from build123d import *

# Parameters (mm, degrees)
BOSS_EXTRUDE1_DEPTH = 29.972
CUT_EXTRUDE1_REACH  = 70.705
SKETCH2_R           = 19.939


with BuildPart() as part:
    # Sketch1 → Boss-Extrude1 (new body, symmetric)
    with BuildSketch(Plane.XY):
        Polygon((0, 0), (0, 59.944), (35.052, 59.944), (109.982, 0), align=None)
    extrude(amount=BOSS_EXTRUDE1_DEPTH, both=True)

    # Cut-Extrude1: up to this face of the body (flat: up to its plane)
    cut_extrude1_end = Plane(part.part.faces().sort_by_distance((54.991, 0, 0))[0])
    # Sketch2 → Cut-Extrude1 (cut, up to the picked face)
    with BuildSketch(Plane(origin=(42.919804878, 53.649756098, 0), x_dir=(0.780868809, -0.624695048, 0), z_dir=(0.624695048, 0.780868809, 0)), mode=Mode.PRIVATE) as cut_extrude1_sk1:
        with Locations((24.4135134, -1.016)):
            Circle(SKETCH2_R)
    cut_extrude1_tool1 = split(extrude(cut_extrude1_sk1.sketch, amount=-CUT_EXTRUDE1_REACH, mode=Mode.PRIVATE), bisect_by=cut_extrude1_end, keep=Keep.BOTH, mode=Mode.PRIVATE)
    add(cut_extrude1_tool1.solids().sort_by_distance((61.983556, 38.398755, 1.016))[0], mode=Mode.SUBTRACT)


solid = part.part
Design review of the part built by this model. Coordinates are the model's own, in mm. Give positions to 0.01 mm unless a question says otherwise; leave off trailing zeros. Loops run counter-clockwise (first coordinate to the right, second up) from the corner with the lowest first, then second, coordinate; pieces in that order, holes last. Notation, with made-up numbers: M 39.25,-31.75 L 73.25,-31.75 A13 cw 73.25,-6.75 Z; hole C 79.25,2 d3. An arc over 180 degrees is marked long. One line per question, with ' | ' between items. Start each with the question number.
1. Add section B-B (z = 3). Write out the cut boundary in (x, y).
2. To check wall thickness, follow L1, parallel to Z at x = 52, y = 26; L2, parallel to Z at x = 42, y = 7; L3, parallel to X at y = 9, z = 3.5. State the ranges of each line that lie inside material, in increasing order.
3. Add section C-C (y = 54). Write out the cut boundary in (x, z).
4. Add section A-A (z = -9). Write out the cut boundary in (x, y).
5. The part is to be moulded in two halves that separate along Z. For faces 1 (the face through (44, 24, 29.972)), 2 (the face through (30.73, 31.22, 0.14)), 3 (the face through (0, 30, 0)), say which applies: released by +Z, released by -Z, zero draft, split by the parting line, or undercut.
6. Insertion check: P1, Ø1.5, axis at y = 27.5, z = -2.5, coming from the -X side; P2, Ø5, axis at y = 33.5, z = -5.5, coming from the +X side; P3, Ø3, axis at x = 93, z = -16, coming from the +Y side. Each pin has a flat end and moves straight along its axis. Give the tip position at first contact, or say it passes through.
7. Add section D-D (z = -24). Write out the cut boundary in (x, y).
Worked out:
1) outline: M 0,0 L 5.86,0 L 46.49,50.79 L 35.05,59.94 L 0,59.94 Z; M 56.67,0 L 109.98,0 L 77.48,26 Z
2) L1: z = -29.97 to -18.92, 20.95 to 29.97 | L2: z = -29.97 to -18.52, 20.55 to 29.97 | L3: x = 0 to 13.13, 63.8 to 98.73
3) outline: M 0,-29.97 L 42.48,-29.97 L 42.48,29.97 L 0,29.97 Z
4) outline: M 0,0 L 9.19,0 L 48.52,49.17 L 35.05,59.94 L 0,59.94 Z; M 53.34,0 L 109.98,0 L 75.45,27.63 Z
5) face 1: released by +Z | face 2: undercut | face 3: zero draft
6) P1: stops at x = 0 | P2: stops at x = 36.29 | P3: stops at y = 14.79
7) outline: M 0,0 L 109.98,0 L 35.05,59.94 L 0,59.94 Z
